from build123d import *

# Parameters (mm, degrees)
F_7_0_7_DIAMETER_HOLE1_D     = 7
F_7_0_7_DIAMETER_HOLE1_DEPTH = 10
M6X1_0_TAPPED_HOLE1_REACH    = 100.969
M6X1_0_TAPPED_HOLE1_BORE_R   = 2.5
CIRPATTERN1_COUNT            = 2
CIRPATTERN1_ANGLE            = 120
CHAMFER1_SIZE                = 1


with BuildPart() as part:
    # Sketch1 → Revolve1 (revolve)
    with BuildSketch(Plane(origin=(0, 0, 0), x_dir=(0, 0, -1), z_dir=(1, 0, 0)), mode=Mode.PRIVATE) as revolve1_sk:
        Polygon((-47.5, 34.5), (-46.5, 34.5), (-46.5, 40.055), (-47.5, 44.5), (-45.5, 44.5), (-44.5, 40.055), (-3, 40.055), (-2, 44.5), (0, 44.5), (-1, 40.055), (-1, 34.5), (0, 34.5), (0, 0), (-47.5, 0), align=None)
    revolve(revolve1_sk.sketch.rotate(Axis((0, 0, 58.930723614), (0, 0, -1)), 90), axis=Axis((0, 0, 58.930723614), (0, 0, -1)))

    # Sketch2 → Cut-Revolve1 (revolve, cut)
    with BuildSketch(Plane(origin=(0, 0, 0), x_dir=(0, 0, -1), z_dir=(1, 0, 0)), mode=Mode.PRIVATE) as cut_revolve1_sk:
        Polygon((-20.5, 17.5), (0, 17.5), (0, 0), (-47.5, 0), (-47.5, 28.5), (-20.5, 28.5), align=None)
    revolve(cut_revolve1_sk.sketch.rotate(Axis((0, 0, 2.983613524), (0, 0, -1)), 90), axis=Axis((0, 0, 2.983613524), (0, 0, -1)), mode=Mode.SUBTRACT)

    # Ø7.0 (7) Diameter Hole1
    with Locations(Plane(origin=(0, 40.055, 0), x_dir=(-1, 0, 0), z_dir=(0, 1, 0))):
        with Locations((0, 23.75)):
            f_7_0_7_diameter_hole1 = Hole(F_7_0_7_DIAMETER_HOLE1_D / 2, depth=F_7_0_7_DIAMETER_HOLE1_DEPTH)

    # M6x1.0 Tapped Hole1 bore → M6x1.0 Tapped Hole1 (cut, up to next)
    with BuildSketch(Plane(origin=(0, 30.055, 0), x_dir=(-1, 0, 0), z_dir=(0, 1, 0)), mode=Mode.PRIVATE) as m6x1_0_tapped_hole1_sk1:
        with Locations((0, 23.75)):
            Circle(M6X1_0_TAPPED_HOLE1_BORE_R)
    m6x1_0_tapped_hole1_tool1 = extrude(m6x1_0_tapped_hole1_sk1.sketch, amount=-M6X1_0_TAPPED_HOLE1_REACH, mode=Mode.PRIVATE) & part.part
    m6x1_0_tapped_hole1 = m6x1_0_tapped_hole1_tool1.solids().sort_by_distance((0, 30.055, 23.75))[0]
    add(m6x1_0_tapped_hole1, mode=Mode.SUBTRACT)

    # CirPattern1: Ø7.0 (7) Diameter Hole1, M6x1.0 Tapped Hole1 ×2 about axis
    cirpattern1_axis = Axis((0, 0, 2.983613524), (0, 0, -1))
    add([f_7_0_7_diameter_hole1.rotate(cirpattern1_axis, i * CIRPATTERN1_ANGLE / (CIRPATTERN1_COUNT - 1)) for i in range(1, CIRPATTERN1_COUNT)], mode=Mode.SUBTRACT)
    add([m6x1_0_tapped_hole1.rotate(cirpattern1_axis, i * CIRPATTERN1_ANGLE / (CIRPATTERN1_COUNT - 1)) for i in range(1, CIRPATTERN1_COUNT)], mode=Mode.SUBTRACT)

    # Chamfer1
    chamfer1_edges = [part.edges().sort_by_distance(p)[0] for p in [
        (-28.5, 0, 47.5),
    ]]
    chamfer(chamfer1_edges, length=CHAMFER1_SIZE)


solid = part.part
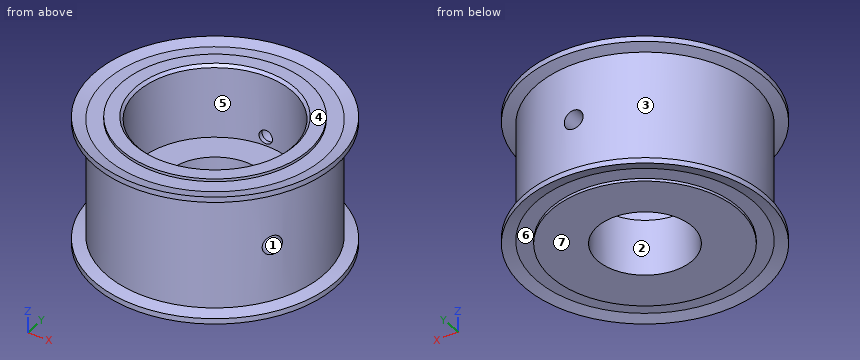
Part model, mm, in its own coordinate system. Face numbers are marked on the shaded views. A direction names the side the tool comes from. Round coordinates to 2 decimals unless told otherwise and drop trailing zeros. Order: outer loops, then holes, each group sorted by start corner. A loop starts at its lowest first (then second) coordinate and runs counter-clockwise, first axis right, second up. Notation, with made-up numbers: (35.25, 86) -> (48.25, 86) arc R22 cw to (48.25, 106) -> close; hole circle Ø4 at (-23.75, 27). An arc over 180 degrees is marked (long way). Put each result on its own line as item: value.
Q1. Band-saw the part on B-B (z = 23.75). Give the cut face in (x, y) (3 decimals).
From the geometry:
outline: (-3.5, 30.055) -> (-3.5, 39.902) arc R40.055 ccw (long way) to (32.806, -22.982) -> (24.278, -18.059) -> (24.778, -17.193) -> (23.337, -16.36) arc R28.5 cw (long way) to (-2.5, 28.39) -> (-2.5, 30.055) -> close; (2.5, 28.39) arc R28.5 cw to (25.837, -12.03) -> (27.278, -12.862) -> (27.778, -11.996) -> (36.306, -16.92) arc R40.055 ccw to (3.5, 39.902) -> (3.5, 30.055) -> (2.5, 30.055) -> close
Q2. Band-saw the part on C-C (z = 38). Give the cut face in (x, y) (3 decimals).
From the geometry:
outline: circle Ø80.11 at (0, 0); hole circle Ø57 at (0, 0)
Q3. Pin check, flat tips, straight feed: pin 1 Ø9 at (x, z) = (0, 23.75) entering from +Y (3 decimals); pin 2 Ø1 at (x, y) = (19.5, 32.5) entering from +Z; pin 3 Ø3 at (x, z) = (0, 23.75) entering from +Y. Stop position of each tip, or through.
From the geometry:
pin 1: stops at y = 40.055
pin 2: stops at z = 46.5
pin 3: stops at y = -28.46
Q4. Tool access for the marked faces 5, 6 and 7: list every direction of +Z, -Z, +X, -X, +Y, -Y with a clear straight run to the whole face (end or side of a thin tool).
From the geometry:
face 5: +Z
face 6: -Z
face 7: -Z, +X, -X, +Y, -Y
Q5. Wall check: line 1 (Z direction, x = 0, y = 33.75); line 2 (Y direction, x = 0, z = 9.75) (3 decimals); line 3 (Z direction, x = -3, y = -35). Give the ranges that are in metal, low to high. Write a range as [from, to].
From the geometry:
line 1: z = [0, 20.25], [27.25, 47.5]
line 2: y = [-40.055, -17.5], [17.5, 40.055]
line 3: z = [1, 46.5]
Q6. Band-saw the part on D-D (x = 0). State how many separate pieces and enclosed holes the cut face has, and give its area (3 significant figures).
From the geometry:
separate pieces: 3
enclosed holes: 0
area: 1,480 mm2
Q7. Pull direction Y, two halves, no side cores. Call the marked faces 1, 2, 3 and 4: pulls with the +Y half, pulls with the -Y half, needs draft (parallel to the pull), parting line crosses it, or undercut.
From the geometry:
face 1: undercut
face 2: undercut
face 3: parting line crosses it
face 4: needs draft
